from build123d import *

# Parameters (mm, degrees)
F0_W     = 38.1
F0_H     = 25.4
F1_DEPTH = 25.4
F3_DEPTH = 12.7
F5_DEPTH = 25.4
F6_DEPTH = 6.35
F4_R     = 6.35
F7_DEPTH = 25.4
F9_DEPTH = 6.35


with BuildPart() as f1:
    # F0 (on Top) → F1 (new body)
    with BuildSketch(Plane.XY):
        with Locations((19.05, 12.7)):
            Rectangle(F0_W, F0_H)
    extrude(amount=F1_DEPTH)

    # F2 (on face) → F3 (cut)
    with BuildSketch(Plane(origin=(0, 0, 0), x_dir=(0, -1, 0), z_dir=(-1, 0, 0))):
        Polygon((-19.05, 25.4), (-25.4, 25.4), (-25.4, 19.05), align=None)
        Polygon((0, 19.05), (0, 25.4), (-6.35, 25.4), align=None)
    extrude(amount=-F3_DEPTH, mode=Mode.SUBTRACT)

    # F4 (on face) → F5 (cut)
    with BuildSketch(Plane.XZ):
        with BuildLine():
            ThreePointArc((28.575, 19.05), (35.3101920908, 16.2601920908), (38.1, 9.525))
            Line((38.1, 9.525), (38.1, 25.4))
            Line((38.1, 25.4), (12.7, 25.4))
            Line((12.7, 25.4), (12.7, 19.05))
            Line((12.7, 19.05), (28.575, 19.05))
        make_face()
        with BuildLine():
            Line((38.1, 0), (38.1, 9.525))
            ThreePointArc((38.1, 9.525), (35.3101920908, 2.7898079092), (28.575, 0))
            Line((28.575, 0), (38.1, 0))
        make_face()
    extrude(amount=-F5_DEPTH, mode=Mode.SUBTRACT)

    # F4 (on face) → F6 (cut)
    with BuildSketch(Plane.XZ):
        with BuildLine():
            ThreePointArc((28.575, 0), (19.05, 9.525), (28.575, 19.05))
            Line((28.575, 19.05), (12.7, 19.05))
            Line((12.7, 19.05), (12.7, 0))
            Line((12.7, 0), (28.575, 0))
        make_face()
    extrude(amount=-F6_DEPTH, mode=Mode.SUBTRACT)

    # F4 (on face) → F7 (cut)
    with BuildSketch(Plane.XZ):
        with Locations((28.575, 9.525)):
            Circle(F4_R)
    extrude(amount=-F7_DEPTH, mode=Mode.SUBTRACT)

    # F8 (on face) → F9 (cut)
    with BuildSketch(Plane(origin=(0, 25.4, 0), x_dir=(-1, 0, 0), z_dir=(0, 1, 0))):
        with BuildLine():
            ThreePointArc((-28.575, 19.05), (-21.8398079092, 16.2601920908), (-19.05, 9.525))
            ThreePointArc((-19.05, 9.525), (-21.8398079092, 2.7898079092), (-28.575, 0))
            Line((-28.575, 0), (-12.7, 0))
            Line((-12.7, 0), (-12.7, 19.05))
            Line((-12.7, 19.05), (-28.575, 19.05))
        make_face()
    extrude(amount=-F9_DEPTH, mode=Mode.SUBTRACT)


solid = f1.part
Input: part model. Units: mm. Frame: model coordinates. A direction names the side the tool comes from. Coordinates: 2 decimals unless noted, no trailing zeros. Loops run counter-clockwise (first coordinate to the right, second up) from the corner with the lowest first, then second, coordinate; pieces in that order, holes last.
(1) Pull-direction query (Z, two-part tool) for faces 4 (the face through (6, 13, 25.4)), 5 (the face through (6, 0, 9)), 6 (the face through (22.23, 12.52, 9.8)), 7 (the face through (11, 13, 0)); classes: released by +Z, released by -Z, zero draft, split by the parting line, or undercut.
(2) Section A-A on y = 3. Return the cut outline in (x, z) (3 decimals), then the cut area to 3 significant figures.
(3) Section C-C on x = 24. Return the cut outline in (y, z).
(4) Section B-B on z = 12.25. Return the cut outline in (x, y), then the cut area to 3 significant figures.
(5) Material intervals for probe 1 along X at (y, z) = (3.25, 10); probe 2 along Z at (x, y) = (15, 7); probe 3 along X at (y, z) = (21, 20), sorted ascending.
(6) First-contact query: pin 1 Ø5 at (x, z) = (17, 13) entering from +Y; pin 2 Ø1 at (x, z) = (27, 3.5) entering from -Y; pin 3 Ø3 at (y, z) = (20.5, 14) entering from +X; pin 4 Ø4 at (x, y) = (17.5, 15.5) entering from +Z. Flat tips, straight axial feed; report the tip coordinate or a pass-through.
(7) Section D-D on y = 7.5. Return the cut outline in (x, z) (3 decimals).
(8) Set-up query: faces 1 (the face through (6, 25.4, 9)), 2 (the face through (12.7, 13, 21)), 3 (the face through (21, 13, 19.05)). Return all of +Z, -Z, +X, -X, +Y, -Y with unobstructed straight access to the full face (end or side cutting, diameter ignored); none if empty.
Data:
1. face 4: released by +Z
1. face 5: zero draft
1. face 6: undercut
1. face 7: released by -Z
2. outline: (0, 0) - (12.7, 0) - (12.7, 22.05) - (0, 22.05) - close; circle Ø19.05 at (28.575, 9.525); hole circle Ø12.7 at (28.575, 9.525)
2. area: 438 mm2
3. outline: (0, 1.17) - (6.35, 1.17) - (6.35, 0) - (19.05, 0) - (19.05, 1.17) - (25.4, 1.17) - (25.4, 5.12) - (0, 5.12) - close; (0, 13.93) - (25.4, 13.93) - (25.4, 17.88) - (19.05, 17.88) - (19.05, 19.05) - (6.35, 19.05) - (6.35, 17.88) - (0, 17.88) - close
4. outline: (0, 0) - (12.7, 0) - (12.7, 6.35) - (19.45, 6.35) - (19.45, 0) - (22.84, 0) - (22.84, 25.4) - (19.45, 25.4) - (19.45, 19.05) - (12.7, 19.05) - (12.7, 25.4) - (0, 25.4) - close; (34.31, 0) - (37.7, 0) - (37.7, 25.4) - (34.31, 25.4) - close
4. area: 581 mm2
5. probe 1: x = 0 to 12.7, 19.06 to 22.24, 34.91 to 38.09
5. probe 2: z = 0 to 19.05
5. probe 3: x = 0 to 12.7
6. pin 1: stops at y = 19.05
6. pin 2: stops at y = 0
6. pin 3: stops at x = 37.62
6. pin 4: stops at z = 19.05
7. outline: (0, 0) - (28.575, 0) arc R9.525 ccw to (28.575, 19.05) - (12.7, 19.05) - (12.7, 25.4) - (0, 25.4) - close; hole circle Ø12.7 at (28.575, 9.525)
8. face 1: +Z, -Z, +X, -X, +Y
8. face 2: +Z
8. face 3: +Z, +X, +Y, -Y
